Model file for the job. Use its own axes, mm. A direction names the side the tool comes from. Round coordinates to 2 decimals unless told otherwise and drop trailing zeros. Order: outer loops, then holes, each group sorted by start corner. A loop starts at its lowest first (then second) coordinate and runs counter-clockwise, first axis right, second up. Notation, with made-up numbers: (62.5, 16) -> (108.5, 16) arc R12 cw to (108.5, 26) -> close; hole circle Ø1 at (79.25, 81.25). An arc over 180 degrees is marked (long way). Use CSV: the item, a comma, the result in double quotes.
```python
from build123d import *

# Parameters (mm, degrees)
SKETCH1_W           = 7.5
SKETCH1_H           = 18.75
BOSS_EXTRUDE1_DEPTH = 3.65
FILLET1_R           = 2.4
FILLET2_R           = 1
CUT_EXTRUDE1_DEPTH  = 0.2
SKETCH3_R           = 0.974780227
SKETCH3_R_2         = 0.962549202
BOSS_EXTRUDE2_DEPTH = 6.2


with BuildPart() as part:
    # Sketch1 → Boss-Extrude1 (new body)
    with BuildSketch(Plane(origin=(0, 0, 0), x_dir=(1, 0, 0), z_dir=(0, 1, 0))):
        with Locations((-16.912251656, 9.375)):
            Rectangle(SKETCH1_W, SKETCH1_H)
    extrude(amount=BOSS_EXTRUDE1_DEPTH)

    # Fillet1
    fillet1_edges = [part.edges().sort_by_distance(p)[0] for p in [
        (-20.662251656, 1.825, -18.75),
        (-13.162251656, 1.825, -18.75),
    ]]
    fillet(fillet1_edges, radius=FILLET1_R)

    # Fillet2
    fillet2_edges = [part.edges().sort_by_distance(p)[0] for p in [
        (-20.662251656, 0, -8.175),
        (-20.662251656, 3.65, -8.175),
        (-16.912251656, 0, -18.75),
        (-13.865195381, 0, -18.047056275),
        (-19.95930793, 0, -18.047056275),
        (-16.912251656, 3.65, -18.75),
        (-13.865195381, 3.65, -18.047056275),
        (-19.95930793, 3.65, -18.047056275),
        (-13.162251656, 3.65, -8.175),
        (-13.162251656, 0, -8.175),
    ]]
    fillet(fillet2_edges, radius=FILLET2_R)

    # Sketch2 → Cut-Extrude1 (cut)
    with BuildSketch(Plane(origin=(0, 3.65, 0), x_dir=(1, 0, 0), z_dir=(0, 1, 0))):
        Polygon((-19.47000828, 10.03416357), (-19.47000828, 10.207240493), (-18.623854434, 10.207240493), (-18.623854434, 10.03416357), (-18.950777511, 10.03416357), (-18.950777511, 8.707240493), (-19.143085203, 8.707240493), (-19.143085203, 10.03416357), align=None)
        Polygon((-18.431546742, 10.207240493), (-17.546931357, 10.207240493), (-17.546931357, 10.03416357), (-18.239239049, 10.03416357), (-18.239239049, 9.611086647), (-17.546931357, 9.611086647), (-17.546931357, 9.438009724), (-18.239239049, 9.438009724), (-18.239239049, 8.880317416), (-17.546931357, 8.880317416), (-17.546931357, 8.707240493), (-18.431546742, 8.707240493), align=None)
        Polygon((-17.373854434, 8.707240493), (-17.173433761, 10.207240493), (-17.097712607, 10.207240493), (-16.528902511, 9.014932801), (-15.960092415, 10.207240493), (-15.883169338, 10.207240493), (-15.681546742, 8.707240493), (-15.87235203, 8.707240493), (-16.005765492, 9.764932801), (-16.492544338, 8.707240493), (-16.565260684, 8.707240493), (-17.050537126, 9.764932801), (-17.183349626, 8.707240493), align=None)
        with BuildLine():
            Line((-15.412315972, 10.207240493), (-15.104924145, 10.207240493))
            add(Edge.make_bspline(
                [(-15.104924145, 10.207240493), (-15.084590431, 10.207229415), (-15.045621744, 10.207208186), (-14.989736478, 10.205769609), (-14.939035959, 10.204527998), (-14.893445271, 10.202141516), (-14.853068216, 10.198872492), (-14.817890297, 10.195028512), (-14.787873744, 10.190705096), (-14.769771411, 10.186796384), (-14.761474626, 10.185004916)],
                knots=[0, 0, 0, 0, 6.0998e-05, 0.000116901, 0.000167704, 0.00021314, 0.00025384, 0.000289212, 0.000319299, 0.000344757, 0.000344757, 0.000344757, 0.000344757], degree=3))
            add(Edge.make_bspline(
                [(-14.761474626, 10.185004916), (-14.749794935, 10.182001417), (-14.726754486, 10.176076436), (-14.693817305, 10.163863296), (-14.662564371, 10.14998558), (-14.633102385, 10.134199208), (-14.60573229, 10.115966796), (-14.579863591, 10.096157565), (-14.55629197, 10.073769594), (-14.534209882, 10.049888971), (-14.51483493, 10.023970245), (-14.497474918, 9.996890427), (-14.483086108, 9.96825619), (-14.47126094, 9.938174045), (-14.462016779, 9.906800832), (-14.455367321, 9.874036593), (-14.451371733, 9.839953174), (-14.450978032, 9.816726583), (-14.450777511, 9.804896743)],
                knots=[0, 0, 0, 0, 3.6158e-05, 7.1328e-05, 0.000105224, 0.000138702, 0.000171454, 0.00020379, 0.000236316, 0.000268858, 0.00030125, 0.000333261, 0.000365243, 0.000397216, 0.000430113, 0.000463231, 0.000497409, 0.000532886, 0.000532886, 0.000532886, 0.000532886], degree=3))
            add(Edge.make_bspline(
                [(-14.450777511, 9.804896743), (-14.450982431, 9.793067454), (-14.451386495, 9.769742405), (-14.455356851, 9.735455231), (-14.462012335, 9.702622928), (-14.470985169, 9.671100454), (-14.482777462, 9.641083852), (-14.496868277, 9.612319712), (-14.513901371, 9.585133925), (-14.533346655, 9.559337792), (-14.55530593, 9.535327744), (-14.579460944, 9.513194915), (-14.606129209, 9.493325844), (-14.635037209, 9.475363904), (-14.666084216, 9.458994121), (-14.699582563, 9.444914312), (-14.735382799, 9.432916973), (-14.76022897, 9.426537659), (-14.772892895, 9.423286166)],
                knots=[0, 0, 0, 0, 3.5477e-05, 6.9954e-05, 0.000103367, 0.000135891, 0.000168143, 0.000199991, 0.000231842, 0.000264234, 0.000296777, 0.000329319, 0.000362372, 0.000396389, 0.000431334, 0.000467554, 0.000505277, 0.000544492, 0.000544492, 0.000544492, 0.000544492], degree=3))
            add(Edge.make_bspline(
                [(-14.772892895, 9.423286166), (-14.782187231, 9.421271087), (-14.802462631, 9.416875234), (-14.836108437, 9.412301035), (-14.875312671, 9.40855358), (-14.920199238, 9.405293226), (-14.970584149, 9.402554499), (-15.026690891, 9.4009242), (-15.0883915, 9.39960867), (-15.13146575, 9.3995689), (-15.153902511, 9.399548185)],
                knots=[0, 0, 0, 0, 2.8522e-05, 6.222e-05, 0.000101776, 0.00014667, 0.000197223, 0.000253141, 0.000315052, 0.000382361, 0.000382361, 0.000382361, 0.000382361], degree=3))
            Line((-15.153902511, 9.399548185), (-15.22000828, 9.399548185))
            Line((-15.22000828, 9.399548185), (-15.22000828, 8.707240493))
            Line((-15.22000828, 8.707240493), (-15.412315972, 8.707240493))
            Line((-15.412315972, 8.707240493), (-15.412315972, 10.207240493))
        make_face()
        with BuildLine():
            Line((-15.22000828, 10.03416357), (-15.22000828, 9.572024147))
            Line((-15.22000828, 9.572024147), (-15.003662126, 9.569620301))
            add(Edge.make_bspline(
                [(-15.003662126, 9.569620301), (-14.991442118, 9.569781438), (-14.96789801, 9.570091898), (-14.933922023, 9.571169852), (-14.90267133, 9.573360722), (-14.874085566, 9.575915893), (-14.848106984, 9.579498254), (-14.824852537, 9.583969214), (-14.804123942, 9.58899258), (-14.780420498, 9.596890423), (-14.753888196, 9.609222279), (-14.72568146, 9.628038142), (-14.700818195, 9.650540527), (-14.680284887, 9.67702579), (-14.663760532, 9.706207338), (-14.651477561, 9.737397026), (-14.644525179, 9.770537082), (-14.643569262, 9.793147018), (-14.643085203, 9.804596262)],
                knots=[0, 0, 0, 0, 3.6664e-05, 7.0639e-05, 0.00010196, 0.000130633, 0.000156725, 0.000180592, 0.000201654, 0.000220658, 0.000255475, 0.00028906, 0.000322027, 0.000355628, 0.000389134, 0.000422335, 0.000455809, 0.000490148, 0.000490148, 0.000490148, 0.000490148], degree=3))
            add(Edge.make_bspline(
                [(-14.643085203, 9.804596262), (-14.643572758, 9.815645957), (-14.644539806, 9.837562612), (-14.65152853, 9.869796434), (-14.663817169, 9.900371212), (-14.680368439, 9.929142837), (-14.700481342, 9.955440534), (-14.724306032, 9.978063055), (-14.751268987, 9.996551957), (-14.776440979, 10.008393772), (-14.798885683, 10.016100206), (-14.818667462, 10.020627198), (-14.841014829, 10.024859872), (-14.866066555, 10.028488465), (-14.893845944, 10.031105466), (-14.924319512, 10.03278413), (-14.957376784, 10.034099627), (-14.980323278, 10.034141709), (-14.992243857, 10.03416357)],
                knots=[0, 0, 0, 0, 3.314e-05, 6.5732e-05, 9.8374e-05, 0.000131619, 0.000165036, 0.000197343, 0.000229764, 0.000262694, 0.000280463, 0.000300869, 0.000323499, 0.000348698, 0.000376774, 0.000407176, 0.000440251, 0.000476009, 0.000476009, 0.000476009, 0.000476009], degree=3))
            Line((-14.992243857, 10.03416357), (-15.22000828, 10.03416357))
        make_face(mode=Mode.SUBTRACT)
    extrude(amount=-CUT_EXTRUDE1_DEPTH, mode=Mode.SUBTRACT)

    # Sketch3 → Boss-Extrude2 (add)
    with BuildSketch(Plane.XY):
        with Locations((-18.59951473, 1.812377858)):
            Circle(SKETCH3_R)
        with Locations((-15.301212194, 1.766139972)):
            Circle(SKETCH3_R_2)
    extrude(amount=BOSS_EXTRUDE2_DEPTH)


solid = part.part
```
Q1. Which spindle directions (+Z, -Z, +X, -X, +Y, -Y) get a long thin tool onto all of the face, cutting with end or side? Do faces 1 (the flat face through (-19, 2, 6.2)), 2 (the cylindrical face through (-19.573, 1.855, 3.057)). Say none if no direction does.
From the geometry:
face 1,"+Z, +X, -X, +Y, -Y"
face 2,"+Z"
Q2. Cut at B-B (y = 2.2). Give the cut face in (x, z), plus the area to 3 significant figures.
From the geometry:
outline,"(-20.66, -16.35) arc R2.4 ccw to (-18.26, -18.75) -> (-15.56, -18.75) arc R2.4 ccw to (-13.16, -16.35) -> (-13.16, 0) -> (-14.44, 0) -> (-14.44, 6.2) -> (-16.16, 6.2) -> (-16.16, 0) -> (-17.71, 0) -> (-17.71, 6.2) -> (-19.49, 6.2) -> (-19.49, 0) -> (-20.66, 0) -> close"
area,"160 mm²"
Q3. Probe line 1 along X through (y, z) = (1.6, 2.25); line 2 along Z through (x, y) = (-16.5, 2.75); line 3 along X through (y, z) = (2.7, -4.5). List the from-to ranges inside material, lowest first.
From the geometry:
line 1,"x = -19.55 to -17.65, -16.25 to -14.35"
line 2,"z = -18.74 to 0"
line 3,"x = -20.66 to -13.16"
Q4. Pin check, flat tip, straight feed: pin 1 (2 mm diameter, centred on x = -19.5, y = 3, fed in from -Z). Stop position of the tip, or through.
From the geometry:
pin 1,"stops at z = -18.73"
Q5. Cut at C-C (y = 3.15). Give the cut face in (x, z), plus the area to 3 significant figures.
From the geometry:
outline,"(-20.53, -16.35) arc R2.27 ccw to (-18.26, -18.62) -> (-15.56, -18.62) arc R2.27 ccw to (-13.3, -16.35) -> (-13.3, 0) -> (-20.53, 0) -> close"
area,"132 mm²"
Q6. Cut at A-A (z = -7.25). Give the cut face in (x, y).
From the geometry:
outline,"(-20.66, 1) arc R1 ccw to (-19.66, 0) -> (-14.16, 0) arc R1 ccw to (-13.16, 1) -> (-13.16, 2.65) arc R1 ccw to (-14.16, 3.65) -> (-19.66, 3.65) arc R1 ccw to (-20.66, 2.65) -> close"
